Verification items for this drawing (mm, ordinates from the low corner). Coordinates: 2 decimals unless noted, no trailing zeros. Write each loop counter-clockwise with the first axis right and the second up, starting at its lowest first coordinate (ties: lowest second). Pieces come first, ordered by that corner, then holes. Notation, with made-up numbers: (68, 44) -> (75, 44) arc R33 cw to (75, 74) -> close; hole circle Ø10 at (19.5, 71). An arc over 180 degrees is marked (long way). Use CSV: the item, a comma, the result in double quotes.
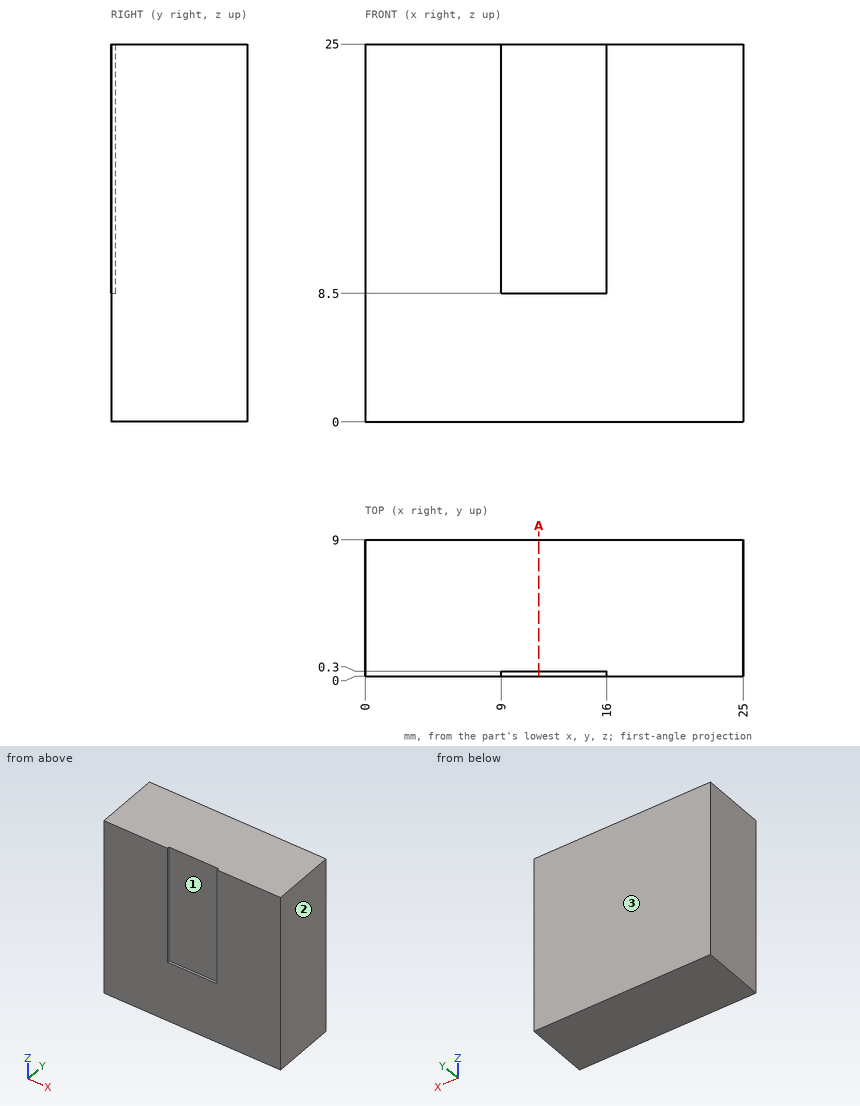
1) Cross-section at A-A (x = 11.5). Record the boundary of the cut face in (y, z), plus the area to 3 significant figures.
Return value:
outline,"(0, 0) -> (9, 0) -> (9, 25) -> (0.3, 25) -> (0.3, 8.5) -> (0, 8.5) -> close"
area,"220 mm2"
2) Mould release check, pull along X, two halves, no side actions. Record for the marked faces 1, 2 and 3: released by +X, released by -X, zero draft, split by the parting line, or undercut.
Return value:
face 1,"undercut"
face 2,"released by +X"
face 3,"zero draft"
3) Scan line: L1, parallel to Y at x = 12, z = 21.25. Record every from-to range of solid material in increasing order.
Return value:
L1,"0.3 to 9"
